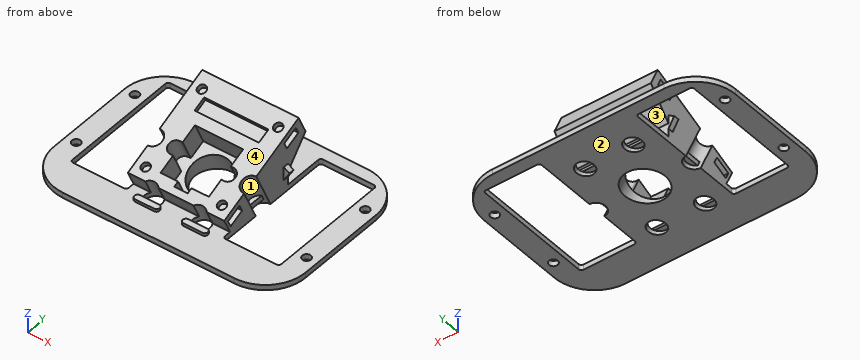
```python
from build123d import *

# Parameters (mm, degrees)
PAD047_DEPTH      = 2
PAD048_DEPTH      = 18
PAD048_DEPTH_BACK = 18
SKETCH145_W       = 21
SKETCH145_H       = 46.5
POCKET061_DEPTH   = 2
FILLET010_R       = 1
POCKET062_DEPTH   = 36
SKETCH147_R       = 3.2
SKETCH147_R_2     = 7.5
POCKET063_DEPTH   = 40
SKETCH148_R       = 3.2
POCKET064_DEPTH   = 16
SKETCH149_R       = 1.6
POCKET065_DEPTH   = 8
POCKET066_DEPTH   = 7
POCKET067_DEPTH   = 7
POCKET068_DEPTH   = 9.5
SKETCH153_W       = 24
SKETCH153_H       = 5
POCKET069_DEPTH   = 1.5
PAD049_DEPTH      = 2
PAD050_DEPTH      = 1
SKETCH156_W       = 5
SKETCH156_H       = 2
PAD051_DEPTH      = 15
SKETCH157_R       = 1.6
POCKET070_DEPTH   = 5


with BuildPart() as part:
    # Sketch143 → Pad047 (new body)
    with BuildSketch(Plane.XY.offset(42)):
        with BuildLine():
            ThreePointArc((10, 0.35), (14.3933982822, -10.2566017178), (25, -14.65))
            Line((25, -14.65), (89, -14.65))
            ThreePointArc((89, -14.65), (99.6066017178, -10.2566017178), (104, 0.35))
            Line((104, 34.05), (104, 0.35))
            ThreePointArc((104, 34.05), (99.6066017178, 44.6566017178), (89, 49.05))
            Line((25, 49.05), (89, 49.05))
            ThreePointArc((25, 49.05), (14.3933982822, 44.6566017178), (10, 34.05))
            Line((10, 34.05), (10, 0.35))
        make_face()
    extrude(amount=PAD047_DEPTH)

    # Sketch144 → Pad048 (join, two sides)
    with BuildSketch(Plane.YZ.offset(57)) as pad048_sk:
        Polygon((-14.65, 44), (49.05, 44), (49.05, 72.9546061157), align=None)
    extrude(amount=PAD048_DEPTH)
    extrude(pad048_sk.sketch, amount=-PAD048_DEPTH_BACK)

    # Sketch145 (on Face8 of Pad048) → Pocket061 (cut)
    with BuildSketch(Plane.XY.offset(44)):
        with Locations((85.5, 21.25)):
            Rectangle(SKETCH145_W, SKETCH145_H)
        with Locations((28.5, 21.25)):
            Rectangle(SKETCH145_W, SKETCH145_H)
    extrude(amount=-POCKET061_DEPTH, mode=Mode.SUBTRACT)

    # Fillet010
    fillet010_edges = [part.edges().sort_by_distance(p)[0] for p in [
        (75, 44.5, 43),
        (96, 44.5, 43),
        (75, -2, 43),
        (96, -2, 43),
        (18, -2, 43),
        (39, -2, 43),
        (39, 44.5, 43),
        (18, 44.5, 43),
    ]]
    fillet(fillet010_edges, radius=FILLET010_R)

    # Sketch146 (on Face31 of Fillet010) → Pocket062 (cut)
    with BuildSketch(Plane.YZ.offset(75)):
        Polygon((-14.65, 44), (1.35, 44), (-1.3897355414, 50.0274055634), align=None)
        Polygon((34.1145443428, 66.1657484122), (37.4249736451, 58.8828192052), (29.05, 49), (29.05, 44), (49.05, 44), (49.05, 72.9546061157), align=None)
    extrude(amount=-POCKET062_DEPTH, mode=Mode.SUBTRACT)

    # Sketch147 (on Face33 of Pocket062) → Pocket063 (cut)
    with BuildSketch(Plane(origin=(0, -19.0839356545, 41.9845704801), x_dir=(1, 0, 0), z_dir=(0, -0.4138036628, 0.9103661509))):
        with Locations((39, 33)):
            Circle(SKETCH147_R)
        with Locations((48, 17.4115427319)):
            Circle(SKETCH147_R)
        with Locations((66, 17.4115427319)):
            Circle(SKETCH147_R)
        with Locations((75, 33)):
            Circle(SKETCH147_R)
        with Locations((57, 33)):
            Circle(SKETCH147_R_2)
    extrude(amount=-POCKET063_DEPTH, mode=Mode.SUBTRACT)

    # Sketch148 (on Face33 of Pocket062) → Pocket064 (cut)
    with BuildSketch(Plane(origin=(0, -11.6354697243, 25.5979797643), x_dir=(1, 0, 0), z_dir=(0, -0.4138036628, 0.9103661509))):
        with Locations((48, 48.5884572681)):
            Circle(SKETCH148_R)
        with Locations((66, 48.5884572681)):
            Circle(SKETCH148_R)
    extrude(amount=-POCKET064_DEPTH, mode=Mode.SUBTRACT)

    # Sketch149 (on Face41 of Pocket064) → Pocket065 (cut)
    with BuildSketch(Plane(origin=(0, -19.0839356545, 41.9845704801), x_dir=(1, 0, 0), z_dir=(0, -0.4138036628, 0.9103661509))):
        with Locations((42.75, 53)):
            Circle(SKETCH149_R)
        with Locations((71.25, 53)):
            Circle(SKETCH149_R)
        with Locations((71.25, 23.5)):
            Circle(SKETCH149_R)
        with Locations((42.75, 23.5)):
            Circle(SKETCH149_R)
    extrude(amount=-POCKET065_DEPTH, mode=Mode.SUBTRACT)

    # Sketch150 (on Face47 of Pocket065) → Pocket066 (cut)
    with BuildSketch(Plane.YZ.offset(75)):
        Polygon((0.4061777641, 48.6468132655), (5.8683746693, 51.1296352423), (7.1097856577, 48.3985367897), (1.6475887524, 45.9157148129), align=None)
        Polygon((27.2619792149, 60.8540213179), (32.7241761202, 63.3368432946), (33.9655871086, 60.605744842), (28.5033902033, 58.1229228652), align=None)
    extrude(amount=-POCKET066_DEPTH, mode=Mode.SUBTRACT)

    # Sketch151 (on Face47 of Pocket065) → Pocket067 (cut)
    with BuildSketch(Plane.YZ.offset(39)):
        Polygon((0.4061777641, 48.6468132655), (5.8683746693, 51.1296352423), (7.1097856577, 48.3985367897), (1.6475887524, 45.9157148129), align=None)
        Polygon((27.2619792149, 60.8540213179), (32.7241761202, 63.3368432946), (33.9655871086, 60.605744842), (28.5033902033, 58.1229228652), align=None)
    extrude(amount=POCKET067_DEPTH, mode=Mode.SUBTRACT)

    # Sketch152 (on Face41 of Pocket067) → Pocket068 (cut)
    with BuildSketch(Plane(origin=(0, -19.0839356545, 41.9845704801), x_dir=(1, 0, 0), z_dir=(0, -0.4138036628, 0.9103661509))):
        with BuildLine():
            Line((48, 42), (66, 42))
            Line((66, 42), (66, 35.5))
            Line((66, 35.5), (67, 35.5))
            ThreePointArc((67, 30.5), (69.5, 33), (67, 35.5))
            Line((67, 30.5), (66, 30.5))
            Line((66, 30.5), (66, 24))
            Line((66, 24), (59.5, 24))
            Line((59.5, 24), (59.5, 22))
            Line((59.5, 22), (54.5, 22))
            Line((54.5, 22), (54.5, 24))
            Line((54.5, 24), (48, 24))
            Line((48, 24), (48, 30.5))
            Line((48, 30.5), (47, 30.5))
            ThreePointArc((47, 35.5), (44.5, 33), (47, 30.5))
            Line((47, 35.5), (48, 35.5))
            Line((48, 35.5), (48, 42))
        make_face()
    extrude(amount=-POCKET068_DEPTH, mode=Mode.SUBTRACT)

    # Sketch153 (on Face41 of Pocket068) → Pocket069 (cut)
    with BuildSketch(Plane(origin=(0, -19.0839356545, 41.9845704801), x_dir=(1, 0, 0), z_dir=(0, -0.4138036628, 0.9103661509))):
        with Locations((57, 48.5)):
            Rectangle(SKETCH153_W, SKETCH153_H)
    extrude(amount=-POCKET069_DEPTH, mode=Mode.SUBTRACT)

    # Sketch154 → Pad049 (join)
    with BuildSketch(Plane.XZ.offset(-29)):
        Polygon((39, 47), (39, 52), (36.8349364905, 50.75), align=None)
        Polygon((75, 52), (75, 47), (77.1650635095, 50.75), align=None)
    extrude(amount=PAD049_DEPTH)

    # Sketch155 (on Face39 of Pad049) → Pad050 (join)
    with BuildSketch(Plane.XY.offset(44)):
        with BuildLine():
            ThreePointArc((44.5, -2.5), (43.3, -3.7), (44.5, -4.9))
            Line((44.5, -4.9), (51.5, -4.9))
            ThreePointArc((51.5, -4.9), (52.7, -3.7), (51.5, -2.5))
            Line((44.5, -2.5), (51.5, -2.5))
        make_face()
        with BuildLine():
            ThreePointArc((44.5, 31.9), (43.3, 30.7), (44.5, 29.5))
            Line((44.5, 29.5), (51.5, 29.5))
            ThreePointArc((51.5, 29.5), (52.7, 30.7), (51.5, 31.9))
            Line((44.5, 31.9), (51.5, 31.9))
        make_face()
        with BuildLine():
            ThreePointArc((62.5, 31.9), (61.3, 30.7), (62.5, 29.5))
            Line((62.5, 29.5), (69.5, 29.5))
            ThreePointArc((69.5, 29.5), (70.7, 30.7), (69.5, 31.9))
            Line((62.5, 31.9), (69.5, 31.9))
        make_face()
        with BuildLine():
            ThreePointArc((62.5, -2.5), (61.3, -3.7), (62.5, -4.9))
            Line((62.5, -4.9), (69.5, -4.9))
            ThreePointArc((69.5, -4.9), (70.7, -3.7), (69.5, -2.5))
            Line((62.5, -2.5), (69.5, -2.5))
        make_face()
    extrude(amount=PAD050_DEPTH)

    # Sketch156 → Pad051 (join)
    with BuildSketch(Plane.XZ.offset(-11)):
        with Locations((43, 45)):
            Rectangle(SKETCH156_W, SKETCH156_H)
        with Locations((71, 45)):
            Rectangle(SKETCH156_W, SKETCH156_H)
    extrude(amount=-PAD051_DEPTH)

    # Sketch157 (on Face38 of Pad051) → Pocket070 (cut)
    with BuildSketch(Plane.XY.offset(44)):
        with Locations((14, 33.95)):
            Circle(SKETCH157_R)
        with Locations((100, 33.95)):
            Circle(SKETCH157_R)
        with Locations((100, 5.95)):
            Circle(SKETCH157_R)
        with Locations((14, 5.95)):
            Circle(SKETCH157_R)
    extrude(amount=-POCKET070_DEPTH, mode=Mode.SUBTRACT)


solid = part.part
```
The listing builds one solid part. Answer for the finished solid, in the listing's coordinates (mm). Face numbers are marked on the shaded views. A direction names the side the tool comes from. Round coordinates to 2 decimals unless told otherwise and drop trailing zeros. Write each loop counter-clockwise with the first axis right and the second up, starting at its lowest first coordinate (ties: lowest second). Pieces come first, ordered by that corner, then holes. Notation, with made-up numbers: (-28.75, 10) -> (-16.75, 10) arc R36 cw to (-16.75, 49) -> close; hole circle Ø10 at (82.5, -35.75). An arc over 180 degrees is marked (long way). Write item = value, one per line.
1) Given pin 1 (5 mm diameter, centred on x = 72, z = 48.5, fed in from +Y); pin 2 (5.5 mm diameter, centred on y = 4, z = 47.5, fed in from -X); pin 3 (3 mm diameter, centred on x = 62.5, z = 58.5, fed in from -Y), each flat-ended and moving along its own axis, determine where each tip first touches the part or whether it passes through.
Check values:
pin_1 = 30.74
pin_2 = 39
pin_3 = 19.15
2) Which of the six approach directions +Z, -Z, +X, -X, +Y, -Y give full straight-line access (tool end or side, diameter ignored) to the marked faces 3 and 4?
Check values:
face_3 = +X, -X, +Y
face_4 = +Z, +X, -X, -Y
3) Straight lines are drawn through the part: line 1 along Y through (x, z) = (100, 42.75); line 2 along X through (y, z) = (8, 45.25); line 3 along Z through (x, y) = (19, -6). For each, find the intervals that lie inside material, in ascending order. Write a range as [from, to].
Check values:
line_1 = [-9.85, 4.35], [7.55, 32.35], [35.55, 44.25]
line_2 = [39, 48], [66, 75]
line_3 = [42, 44]
4) For a pull along X with two mould halves and no side action, classify the marked faces 1 and 2 as released by +X, released by -X, zero draft, split by the parting line, or undercut.
Check values:
face_1 = undercut
face_2 = zero draft
5) Section A-A on x = 85.5 is taken. Write down the section's boundary in (y, z), plus the area to 3 significant figures.
Check values:
outline = (-14.65, 42) -> (-2, 42) -> (-2, 44) -> (-14.65, 44) -> close; (44.5, 42) -> (49.05, 42) -> (49.05, 44) -> (44.5, 44) -> close
area = 34.4 mm²
